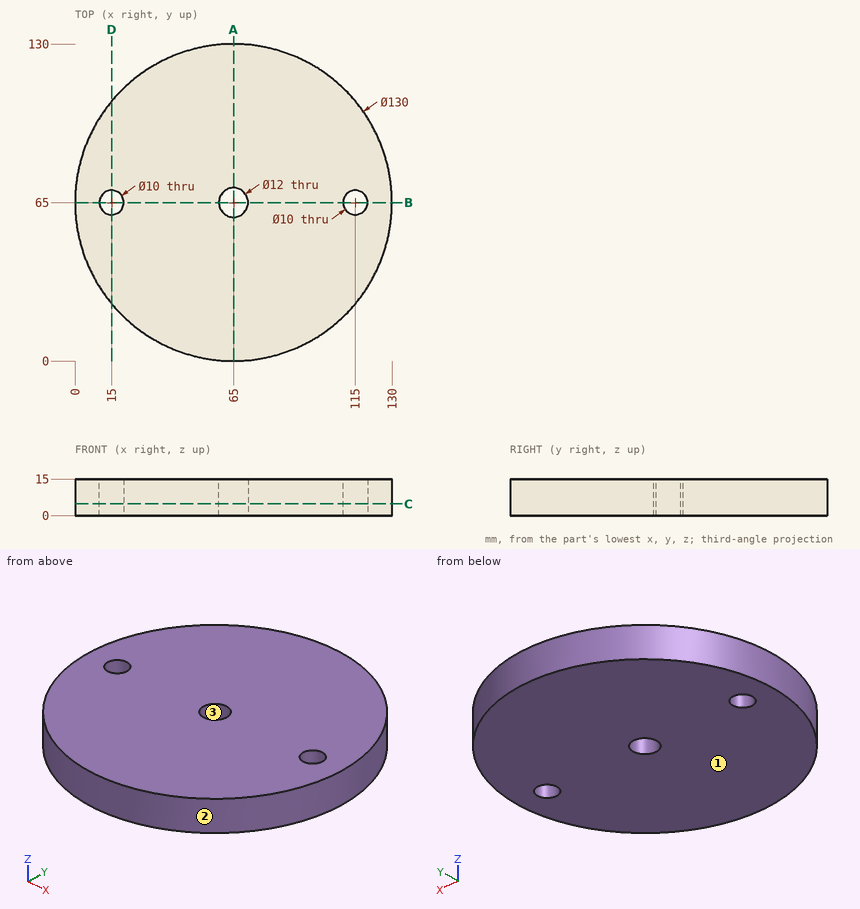
Design review of the part shown in the three views and the two pictorial views. Dimensions are in mm from the part's minimum x, y and z. Round coordinates to 2 decimals unless told otherwise and drop trailing zeros. Loops run counter-clockwise (first coordinate to the right, second up) from the corner with the lowest first, then second, coordinate; pieces in that order, holes last. Notation, with made-up numbers: (60, 77) - (76, 77) arc R18 cw to (76, 82) - close; hole circle Ø7 at (-37.75, -26). An arc over 180 degrees is marked (long way). Answer as CSV lines item,"result".
(1) Insertion check: P1, Ø6, axis at x = 115, z = 6.5, coming from the -Y side; P2, Ø4, axis at x = 99, z = 7, coming from the -Y side; P3, Ø2, axis at x = 28.5, z = 13.5, coming from the +Y side. Each pin has a flat end and moves straight along its axis. Give the tip position at first contact, or say it passes through.
Checked values:
P1,"stops at y = 20.1"
P2,"stops at y = 8.42"
P3,"stops at y = 119.45"
(2) Consider section A-A on x = 65. Give the boundary of the cut face in (y, z), then the cut area to 3 significant figures.
Checked values:
outline,"(0, 0) - (59, 0) - (59, 15) - (0, 15) - close; (71, 0) - (130, 0) - (130, 15) - (71, 15) - close"
area,"1,770 mm2"
(3) Consider section D-D on x = 15. Give the boundary of the cut face in (y, z), then the cut area to 3 significant figures.
Checked values:
outline,"(23.47, 0) - (60, 0) - (60, 15) - (23.47, 15) - close; (70, 0) - (106.53, 0) - (106.53, 15) - (70, 15) - close"
area,"1,100 mm2"
(4) Consider section B-B on y = 65. Give the boundary of the cut face in (x, z).
Checked values:
outline,"(0, 0) - (10, 0) - (10, 15) - (0, 15) - close; (20, 0) - (59, 0) - (59, 15) - (20, 15) - close; (71, 0) - (110, 0) - (110, 15) - (71, 15) - close; (120, 0) - (130, 0) - (130, 15) - (120, 15) - close"
(5) Consider section C-C on z = 4.75. Give the boundary of the cut face in (x, y).
Checked values:
outline,"circle Ø130 at (65, 65); hole circle Ø10 at (15, 65); hole circle Ø12 at (65, 65); hole circle Ø10 at (115, 65)"
(6) Mouldability with a two-part tool opening along Y and no side actions: class the marked faces 1, 2 and 3 as +Y half, -Y half, draft (parallel to the pull), parting line (faces both ways), or undercut.
Checked values:
face 1,"draft"
face 2,"parting line"
face 3,"undercut"
(7) Wall thickness on line 1 (Y direction, x = 65, z = 5.5); line 2 (Y direction, x = 15, z = 10); line 3 (Y direction, x = 84, z = 4.5): over which ranges is each line inside the solid? List them lowest first.
Checked values:
line 1,"y = 0 to 59, 71 to 130"
line 2,"y = 23.47 to 60, 70 to 106.53"
line 3,"y = 2.84 to 127.16"
